```python
from build123d import *

# Parameters (mm, degrees)
SKETCH2_R             = 2.1
BOSS_EXTRUDE1_DEPTH   = 5
BOSS_EXTRUDE1_2_DEPTH = 5
BOSS_EXTRUDE1_3_DEPTH = 5
BOSS_EXTRUDE1_4_DEPTH = 5
SKETCH3_W             = 7.6
SKETCH3_H             = 26
BOSS_EXTRUDE2_DEPTH   = 15
CHAMFER1_SIZE         = 1
CHAMFER1_SIZE2        = 0.577350269
CHAMFER1_PART_2_SIZE  = 1
CHAMFER1_PART_2_SIZE2 = 0.577350269
CHAMFER2_SIZE         = 1
CHAMFER2_SIZE2        = 0.577350269
CHAMFER2_PART_2_SIZE  = 1
CHAMFER2_PART_2_SIZE2 = 0.577350269
SKETCH4_W             = 56.3
SKETCH4_H             = 12
BOSS_EXTRUDE3_DEPTH   = 15
CUT_EXTRUDE1_DEPTH    = 42.151215049
CUT_EXTRUDE2_DEPTH    = 3
CHAMFER7_SIZE         = 2
SKETCH7_W             = 4.3
SKETCH7_H             = 6.3
CUT_EXTRUDE3_DEPTH    = 42.790220148


with BuildPart() as part:
    # Sketch2 → Boss-Extrude1 (new body)
    with BuildSketch(Plane(origin=(0, 0, 0), x_dir=(1, 0, 0), z_dir=(0, 1, 0))):
        with Locations(Location((-24.35, 5, 0), (0, 0, 270))):
            Circle(SKETCH2_R)
    extrude(amount=BOSS_EXTRUDE1_DEPTH)



with BuildPart() as body_2:
    # Sketch2 → Boss-Extrude1 2 (new body)
    with BuildSketch(Plane(origin=(0, 0, 0), x_dir=(1, 0, 0), z_dir=(0, 1, 0))):
        with Locations(Location((-24.35, -5, 0), (0, 0, 270))):
            Circle(SKETCH2_R)
    extrude(amount=BOSS_EXTRUDE1_2_DEPTH)


with BuildPart() as body_3:
    # Sketch2 → Boss-Extrude1 3 (new body)
    with BuildSketch(Plane(origin=(0, 0, 0), x_dir=(1, 0, 0), z_dir=(0, 1, 0))):
        with Locations(Location((24.35, -5, 0), (0, 0, 90))):
            Circle(SKETCH2_R)
    extrude(amount=BOSS_EXTRUDE1_3_DEPTH)


with BuildPart() as body_4:
    # Sketch2 → Boss-Extrude1 4 (new body)
    with BuildSketch(Plane(origin=(0, 0, 0), x_dir=(1, 0, 0), z_dir=(0, 1, 0))):
        with Locations(Location((24.35, 5, 0), (0, 0, 90))):
            Circle(SKETCH2_R)
    extrude(amount=BOSS_EXTRUDE1_4_DEPTH)


with BuildPart() as part_1:
    add(part.part)

    add(body_2.part)  # Boss-Extrude2 merges body 2

    add(body_3.part)  # Boss-Extrude2 merges body 3

    add(body_4.part)  # Boss-Extrude2 merges body 4
    # Sketch3 → Boss-Extrude2 (add)
    with BuildSketch(Plane(origin=(0, 0, 0), x_dir=(1, 0, 0), z_dir=(0, 1, 0))):
        with Locations((-24.35, 2)):
            Rectangle(SKETCH3_W, SKETCH3_H)
        with Locations((24.35, 2)):
            Rectangle(SKETCH3_W, SKETCH3_H)
    extrude(amount=-BOSS_EXTRUDE2_DEPTH)

    # Chamfer1
    chamfer1_edges = [part_1.edges().sort_by_distance(p)[0] for p in [
        (-24.35, 5, 2.9),
    ]]
    chamfer1_side = [part_1.faces().sort_by_distance(p)[0] for p in [
        (-24.35, 2.5, 2.9),
    ]]
    chamfer(chamfer1_edges, length=CHAMFER1_SIZE, length2=CHAMFER1_SIZE2, reference=chamfer1_side[0])

    # Chamfer1 part 2
    chamfer1_part_2_edges = [part_1.edges().sort_by_distance(p)[0] for p in [
        (-24.35, 5, -7.1),
    ]]
    chamfer1_part_2_side = [part_1.faces().sort_by_distance(p)[0] for p in [
        (-24.35, 2.5, -7.1),
    ]]
    chamfer(chamfer1_part_2_edges, length=CHAMFER1_PART_2_SIZE, length2=CHAMFER1_PART_2_SIZE2, reference=chamfer1_part_2_side[0])

    # Chamfer2
    chamfer2_edges = [part_1.edges().sort_by_distance(p)[0] for p in [
        (24.35, 5, -2.9),
    ]]
    chamfer2_side = [part_1.faces().sort_by_distance(p)[0] for p in [
        (24.35, 2.5, -2.9),
    ]]
    chamfer(chamfer2_edges, length=CHAMFER2_SIZE, length2=CHAMFER2_SIZE2, reference=chamfer2_side[0])

    # Chamfer2 part 2
    chamfer2_part_2_edges = [part_1.edges().sort_by_distance(p)[0] for p in [
        (24.35, 5, 7.1),
    ]]
    chamfer2_part_2_side = [part_1.faces().sort_by_distance(p)[0] for p in [
        (24.35, 2.5, 7.1),
    ]]
    chamfer(chamfer2_part_2_edges, length=CHAMFER2_PART_2_SIZE, length2=CHAMFER2_PART_2_SIZE2, reference=chamfer2_part_2_side[0])

    # Sketch4 → Boss-Extrude3 (add)
    with BuildSketch(Plane(origin=(0, 0, 0), x_dir=(1, 0, 0), z_dir=(0, 1, 0))):
        with Locations((0, 21)):
            Rectangle(SKETCH4_W, SKETCH4_H)
    extrude(amount=-BOSS_EXTRUDE3_DEPTH)

    # Sketch5 → Cut-Extrude1 (cut, through all)
    with BuildSketch(Plane.XY.offset(-15)):
        with BuildLine():
            Line((-11.654372972, -6.085786438), (-10.24015941, -4.671572875))
            Line((-10.24015941, -4.671572875), (-8.825945848, -6.085786438))
            ThreePointArc((-8.825945848, -6.085786438), (-10.24015941, -9.5), (-11.654372972, -6.085786438))
        make_face()
        with BuildLine():
            ThreePointArc((11.654372972, -6.085786438), (10.24015941, -9.5), (8.825945848, -6.085786438))
            Line((8.825945848, -6.085786438), (10.24015941, -4.671572875))
            Line((10.24015941, -4.671572875), (11.654372972, -6.085786438))
        make_face()
    extrude(amount=-CUT_EXTRUDE1_DEPTH, mode=Mode.SUBTRACT)

    # Sketch6 → Cut-Extrude2 (cut)
    with BuildSketch(Plane.XY.offset(-15)):
        with BuildLine():
            Line((-6.704625504, -3.964466094), (-10.24015941, -0.428932188))
            Line((-10.24015941, -0.428932188), (-13.775693316, -3.964466094))
            ThreePointArc((-13.775693316, -3.964466094), (-10.24015941, -12.5), (-6.704625504, -3.964466094))
        make_face()
        with BuildLine():
            Line((13.775693316, -3.964466094), (10.24015941, -0.428932188))
            Line((10.24015941, -0.428932188), (6.704625504, -3.964466094))
            ThreePointArc((6.704625504, -3.964466094), (10.24015941, -12.5), (13.775693316, -3.964466094))
        make_face()
    extrude(amount=-CUT_EXTRUDE2_DEPTH, mode=Mode.SUBTRACT)

    # Chamfer7
    chamfer7_edges = [part_1.edges().sort_by_distance(p)[0] for p in [
        (0, -15, -15),
        (28.15, -15, -8),
        (0, -15, -27),
        (24.35, -15, 11),
        (28.15, -7.5, 11),
        (20.55, -15, -2),
        (20.55, -7.5, 11),
        (-20.55, -15, -2),
        (-24.35, -15, 11),
        (-20.55, -7.5, 11),
        (-28.15, -15, -8),
        (-28.15, -7.5, 11),
    ]]
    chamfer(chamfer7_edges, length=CHAMFER7_SIZE)

    # Sketch7 → Cut-Extrude3 (cut, through all)
    with BuildSketch(Plane(origin=(0, 0, 0), x_dir=(1, 0, 0), z_dir=(0, 1, 0))):
        with Locations((19.5, 20.75)):
            Rectangle(SKETCH7_W, SKETCH7_H)
    extrude(amount=-CUT_EXTRUDE3_DEPTH, mode=Mode.SUBTRACT)


solid = part_1.part
```
Design review of the part built by this model. Coordinates are the model's own, in mm. A direction names the side the tool comes from. Coordinates: 2 decimals unless noted, no trailing zeros. Order: outer loops, then holes, each group sorted by start corner. A loop starts at its lowest first (then second) coordinate and runs counter-clockwise, first axis right, second up. Notation, with made-up numbers: M 20,-23.75 L 72,-23.75 A22 cw 72,13.25 Z; hole C 80.25,44 d5. An arc over 180 degrees is marked long. Answer as a JSON object with one key per item and string values. Group by question number.
1) Add section A-A, the plane y = -7.5. Count the separate pieces of the cut face and the enclosed holes in it, then the cut area to 3 significant figures.
2) Add section D-D, the plane z = 5. Write out the cut boundary in (x, y), then the cut area to 3 significant figures.
3) Tool access review of faces 4 (the cylindrical face through (-22.268, 1.972, 4.727)), 5 (the flat face through (0, -14, -16)), 6 (the flat face through (0, -6, -15)), 7 (the flat face through (19, -7, -17.6)): name each direction out of +Z, -Z, +X, -X, +Y, -Y from which nothing blocks a thin tool from reaching the whole face with its end or side.
4) For pin 1 (8 mm diameter, centred on x = -12.5, y = -9, fed in from +Z); pin 2 (5 mm diameter, centred on x = -10.24, y = -7.5, fed in from +Z); pin 3 (12 mm diameter, centred on x = 12.5, z = -7.5, fed in from +Y); pin 4 (19 mm diameter, centred on x = 13.5, z = -1.5, fed in from +Y), all flat-tipped, find the tip position at first contact; note any pin that passes through.
5) Add section C-C, the plane x = 24.35. Write out the cut boundary in (y, z), then the cut area to 3 significant figures.
6) Wall thickness on L1, parallel to X at y = -7.5, z = -24; L2, parallel to X at y = -7.5, z = -22.25; L3, parallel to X at y = -6, z = -3.5: over which ranges is each line inside the solid? List them lowest first.
7) Add section B-B, the plane z = -10.5. Write out the cut boundary in (x, y), then the cut area to 3 significant figures.
8) Mouldability with a two-part tool opening along Y and no side actions: class faces 1 (the flat face through (21.65, -7, -21)), 2 (the flat face through (24, 5, -5)), 3 (the flat face through (12.03, -2.22, -16.48)) as pulls with the +Y half, pulls with the -Y half, needs draft (parallel to the pull), parting line crosses it, or undercut.
Computed values:
{
 "1": {"separate pieces": "3", "enclosed holes": "1", "area": "904 mm^2"},
 "2": {"outline": "M -28.15,-13 L -26.15,-15 L -22.55,-15 L -20.55,-13 L -20.55,0 L -22.25,0 L -22.25,4 L -22.83,5 L -25.87,5 L -26.45,4 L -26.45,0 L -28.15,0 Z; M 20.55,-13 L 22.55,-15 L 26.15,-15 L 28.15,-13 L 28.15,0 L 26.45,0 L 26.45,4 L 25.87,5 L 22.83,5 L 22.25,4 L 22.25,0 L 20.55,0 Z", "area": "261 mm^2"},
 "3": {"face 4": "+Y", "face 5": "+Z, -Y", "face 6": "+Z, +Y, -Y", "face 7": "+Y, -Y"},
 "4": {"pin 1": "stops at z = -15", "pin 2": "stops at z = -18", "pin 3": "passes through", "pin 4": "stops at y = 4.35"},
 "5": {"outline": "M -15,-25 L -13,-27 L 0,-27 L 0,-7.1 L 4,-7.1 L 5,-6.52 L 5,-3.48 L 4,-2.9 L 0,-2.9 L 0,2.9 L 4,2.9 L 5,3.48 L 5,6.52 L 4,7.1 L 0,7.1 L 0,11 L -13,11 L -15,9 Z", "area": "607 mm^2"},
 "6": {"L1": "x = -28.15 to -12.24, -8.24 to 8.24, 12.24 to 28.15", "L2": "x = -28.15 to -12.24, -8.24 to 8.24, 12.24 to 17.35, 21.65 to 28.15", "L3": "x = -28.15 to -20.55, 20.55 to 28.15"},
 "7": {"outline": "M -28.15,-13 L -26.15,-15 L -22.55,-15 L -20.55,-13 L -20.55,0 L -28.15,0 Z; M 20.55,-13 L 22.55,-15 L 26.15,-15 L 28.15,-13 L 28.15,0 L 20.55,0 Z", "area": "220 mm^2"},
 "8": {"face 1": "needs draft", "face 2": "pulls with the +Y half", "face 3": "undercut"}
}
